Input: part model. Units: mm. Frame: model coordinates. Give positions to 0.01 mm unless a question says otherwise; leave off trailing zeros. Order: outer loops, then holes, each group sorted by start corner. A loop starts at its lowest first (then second) coordinate and runs counter-clockwise, first axis right, second up. Notation, with made-up numbers: (-10.75, -23) -> (-1.75, -23) arc R13 cw to (-1.75, 2) -> close; hole circle Ø2 at (29.25, 85.25). An arc over 180 degrees is marked (long way). Use a Markdown table: item, result. Add a question column.
from build123d import *

# Parameters (mm, degrees)
SKETCH1_W           = 86
SKETCH1_H           = 50
BOSS_EXTRUDE1_DEPTH = 1.3
SKETCH2_W           = 1.4
SKETCH2_H           = 25
BOSS_EXTRUDE2_DEPTH = 1.3
SKETCH3_W           = 30
SKETCH3_H           = 1.4
CUT_EXTRUDE1_DEPTH  = 51.971070226
SKETCH4_W           = 86
SKETCH4_H           = 1
BOSS_EXTRUDE3_DEPTH = 1.3


with BuildPart() as part:
    # Sketch1 → Boss-Extrude1 (new body)
    with BuildSketch(Plane(origin=(0, 0, 0), x_dir=(1, 0, 0), z_dir=(0, 1, 0))):
        Rectangle(SKETCH1_W, SKETCH1_H)
    extrude(amount=BOSS_EXTRUDE1_DEPTH)

    # Sketch2 → Boss-Extrude2 (add)
    with BuildSketch(Plane(origin=(0, 1.3, 0), x_dir=(1, 0, 0), z_dir=(0, 1, 0))):
        with Locations((-43.7, 2.5)):
            Rectangle(SKETCH2_W, SKETCH2_H)
        with Locations((43.7, 2.5)):
            Rectangle(SKETCH2_W, SKETCH2_H)
    extrude(amount=-BOSS_EXTRUDE2_DEPTH)

    # Sketch3 → Cut-Extrude1 (cut, through all)
    with BuildSketch(Plane(origin=(0, 1.3, 0), x_dir=(1, 0, 0), z_dir=(0, 1, 0))):
        with Locations((0, 4.3)):
            Rectangle(SKETCH3_W, SKETCH3_H)
    extrude(amount=-CUT_EXTRUDE1_DEPTH, mode=Mode.SUBTRACT)

    # Sketch4 → Boss-Extrude3 (add)
    with BuildSketch(Plane(origin=(0, 0, 0), x_dir=(1, 0, 0), z_dir=(0, 1, 0))):
        with Locations((0, 25.5)):
            Rectangle(SKETCH4_W, SKETCH4_H)
    extrude(amount=BOSS_EXTRUDE3_DEPTH)


solid = part.part
Q1. Section query B-B (x = 7). Return loops of the section in (y, z).
Q2. Section query C-C (z = -21.5). Return loops of the section in (x, y), plus the area to 3 significant figures.
Q3. Section query A-A (y = 1.1). Return loops of the section in (x, z), plus the area to 3 significant figures.
Q4. Ray query, line 1 (Z direction, x = -12, y = 0.25); line 2 (X direction, y = 1.2, z = -18.5). Return the intervals inside material, ascending.
Q5. First-contact query: pin 1 (0.6 mm diameter, centred on y = 0.5, z = -19.5, fed in from -X). Flat tip, straight axial feed; report the tip coordinate or a pass-through.
Solution:
| question | item | result |
|---|---|---|
| 1 | outline | (0, -26) -> (1.3, -26) -> (1.3, -5) -> (0, -5) -> close; (0, -3.6) -> (1.3, -3.6) -> (1.3, 25) -> (0, 25) -> close |
| 2 | outline | (-43, 0) -> (43, 0) -> (43, 1.3) -> (-43, 1.3) -> close |
| 2 | area | 112 mm² |
| 3 | outline | (-44.4, -15) -> (-43, -15) -> (-43, -26) -> (43, -26) -> (43, -15) -> (44.4, -15) -> (44.4, 10) -> (43, 10) -> (43, 25) -> (-43, 25) -> (-43, 10) -> (-44.4, 10) -> close; hole (-15, -5) -> (15, -5) -> (15, -3.6) -> (-15, -3.6) -> close |
| 3 | area | 4,410 mm² |
| 4 | line 1 | z = -26 to -5, -3.6 to 25 |
| 4 | line 2 | x = -43 to 43 |
| 5 | pin 1 | stops at x = -43 |
